Check sheet for the modelled part. Datum: model origin and axes. Units: mm. Face numbers are marked on the shaded views. Round coordinates to 2 decimals unless told otherwise and drop trailing zeros. Loops run counter-clockwise (first coordinate to the right, second up) from the corner with the lowest first, then second, coordinate; pieces in that order, holes last. Notation, with made-up numbers: (24, 64) -> (69, 64) arc R27 ccw to (69, 86) -> close; hole circle Ø3 at (-12, -3). An arc over 180 degrees is marked (long way). One line per item, written item: value. Start each with the question number.
1. Material ranges on L1, parallel to Z at x = -9.5, y = 27.85; L2, parallel to Y at x = -10, z = 12.5; L3, parallel to Y at x = -11.5, z = 5.75, recorded low to high.
2. Cross-section at C-C on z = 18.25. Record the cut outline in (x, y).
3. Cross-section at D-D on x = -16. Record the cut outline in (y, z), then the cut area to 3 significant figures.
4. Cross-section at A-A on z = 10. Record the cut outline in (x, y) (3 decimals).
5. Go/stop test with flat-tipped pins: pin 1 (5 mm diameter, centred on x = -3, z = 17, fed in from +Y); pin 2 (1.5 mm diameter, centred on x = -20, z = 8.5, fed in from -Y); pin 3 (0.6 mm diameter, centred on x = -9, y = 27, fed in from -Z). Record where each tip stops, or that it passes through.
6. Cross-section at B-B on x = -9.5. Record the cut outline in (y, z).
7. Release check for a two-part mould opening along X. For the marked faces 1, 2 and 3 record: +X half, -X half, draft (parallel to the pull), parting line (faces both ways), or undercut.
from build123d import *

# Parameters (mm, degrees)
F1_DEPTH  = 20
F3_DEPTH  = 5
F5_DEPTH  = 5
F8_DEPTH  = 3
F9_DEPTH  = 1
F6_R      = 1.5
F10_DEPTH = 1
F11_R     = 0.4


with BuildPart() as f1:
    # F0 (on Top) → F1 (new body)
    with BuildSketch(Plane.XY):
        with BuildLine():
            ThreePointArc((-24.5367908878, 4.7901871498), (-15.894107733, 19.2970811102), (0, 25))
            Line((0, 25), (0, 26))
            Line((0, 26), (-4, 27.9999999299))
            Line((-4, 27.9999999299), (-5.9999998598, 27.9999999299))
            Line((-5.9999998598, 27.9999999299), (-7.9999998598, 27.9999999299))
            Line((-7.9999998598, 27.9999999299), (-15, 27.9999999299))
            Line((-15, 27.9999999299), (-15, 26))
            Line((-15, 26), (-4.6190696853, 26))
            Line((-4.6190696853, 26), (-4, 25.6904651573))
            ThreePointArc((-4, 25.6904651573), (-19.7484176581, 16.9115345253), (-26, 0))
            Line((-26, 0), (-24.5367908878, 4.7901871498))
        make_face()
    extrude(amount=F1_DEPTH)

    # F2 (on face) → F3 (cut)
    with BuildSketch(Plane.XY.offset(20)):
        Polygon((-15, 26), (-4.6190696853, 26), (-4, 27.9999999299), (-15, 27.9999999299), align=None)
    extrude(amount=-F3_DEPTH, mode=Mode.SUBTRACT)

    # F4 (on face) → F5 (cut)
    with BuildSketch(Plane(origin=(0, 0, 0), x_dir=(1, 0, 0), z_dir=(0, 0, -1))):
        Polygon((-4, -27.9999999299), (-4.6190696853, -26), (-15, -26), (-15, -27.9999999299), align=None)
    extrude(amount=-F5_DEPTH, mode=Mode.SUBTRACT)

    # F7 (on face) → F8 (join)
    with BuildSketch(Plane(origin=(0, 27.9999999299, 0), x_dir=(-1, 0, 0), z_dir=(0, 1, 0))):
        Polygon((11.775, 12), (11.775, 10), (11.775, 8), (13.775, 8), (13.775, 12), align=None)
        Polygon((7.225, 10), (7.225, 12), (5.225, 12), (5.225, 8), (7.225, 8), align=None)
    extrude(amount=F8_DEPTH)

    # F9 (cut): a face of the model
    f9_faces = [f1.faces().sort_by_distance(p)[0] for p in [
        (-9.8095348427, 26, 10),
    ]]
    extrude(f9_faces, amount=-F9_DEPTH, mode=Mode.SUBTRACT)

    # F6 (on face) → F10 (cut)
    with BuildSketch(Plane(origin=(0, 27.9999999299, 0), x_dir=(-1, 0, 0), z_dir=(0, 1, 0))):
        with Locations((9.5, 10)):
            Circle(F6_R)
    extrude(amount=-F10_DEPTH, mode=Mode.SUBTRACT)

    # F11
    f11_edges = [f1.edges().sort_by_distance(p)[0] for p in [
        (-26, 0, 10),
    ]]
    fillet(f11_edges, radius=F11_R)


solid = f1.part
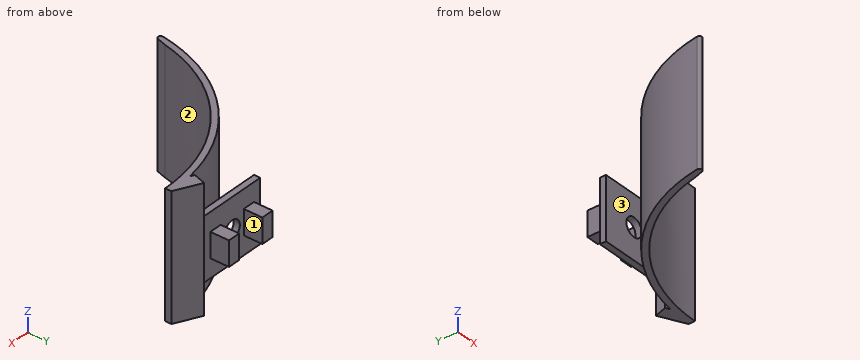
Taken from the geometry:
1. L1: z = 5 to 8.5, 11.5 to 15
1. L2: y = 22.91 to 24, 27 to 28
1. L3: y = 22.2 to 23.32, 27 to 28
2. outline: (-25.76, 3.49) arc R0.4 ccw to (-24.99, 3.32) -> (-24.54, 4.79) arc R25 cw to (0, 25) -> (0, 26) -> (-4, 28) -> (-4.62, 26) -> (-4, 25.69) arc R26 ccw to start
3. outline: (19.21, 0) -> (20.49, 0) -> (20.49, 20) -> (19.21, 20) -> close
3. area: 25.7 mm2
4. outline: (-25.764, 3.492) arc R0.4 ccw to (-24.986, 3.321) -> (-24.537, 4.79) arc R25 cw to (0, 25) -> (0, 26) -> (-4, 28) -> (-5.225, 28) -> (-5.225, 31) -> (-7.225, 31) -> (-7.225, 28) -> (-8, 28) -> (-8, 27) -> (-4.619, 27) -> (-4.619, 26) -> (-4, 25.69) arc R26 ccw to start; (-15, 27) -> (-11, 27) -> (-11, 28) -> (-11.775, 28) -> (-11.775, 31) -> (-13.775, 31) -> (-13.775, 28) -> (-15, 28) -> close
5. pin 1: stops at y = 28
5. pin 2: stops at y = 13.94
5. pin 3: stops at z = 5
6. outline: (23.12, 0) -> (24.2, 0) -> (24.2, 20) -> (23.12, 20) -> close; (27, 5) -> (28, 5) -> (28, 8.5) -> (27, 8.5) -> close; (27, 11.5) -> (28, 11.5) -> (28, 15) -> (27, 15) -> close
7. face 1: undercut
7. face 2: +X half
7. face 3: draft
